Read the model definition and answer for the solid it produces. Units are mm, in the model's axes. Coordinates: 2 decimals unless noted, no trailing zeros. Use one line per item in the form item = value. Start each with the question number.
from build123d import *

# Parameters (mm, degrees)
BASE_FLANGE1_DEPTH = 3.175
SKETCH6_R          = 4.7625
CUT_EXTRUDE1_DEPTH = 140.880281402


# Sheet-metal steps are written as plain solids
with BuildPart() as part:
    # Sketch1 → Base-Flange1 (new body)
    with BuildSketch(Plane(origin=(0, 0, 0), x_dir=(1, 0, 0), z_dir=(0, 1, 0))):
        with BuildLine():
            Line((-69.85, -107.95), (69.85, -107.95))
            ThreePointArc((69.85, -107.95), (83.320384182, -102.370384182), (88.9, -88.9))
            Line((88.9, -88.9), (88.9, 88.9))
            ThreePointArc((88.9, 88.9), (83.320384182, 102.370384182), (69.85, 107.95))
            Line((69.85, 107.95), (-69.85, 107.95))
            ThreePointArc((-69.85, 107.95), (-83.320384182, 102.370384182), (-88.9, 88.9))
            Line((-88.9, 88.9), (-88.9, -88.9))
            ThreePointArc((-88.9, -88.9), (-83.320384182, -102.370384182), (-69.85, -107.95))
        make_face()
    extrude(amount=-BASE_FLANGE1_DEPTH)

    # Sketch6 → Cut-Extrude1 (cut, through all)
    with BuildSketch(Plane(origin=(0, 0, 0), x_dir=(1, 0, 0), z_dir=(0, 1, 0))):
        with Locations(Location((-69.85, -88.9, 0), (0, 0, 270))):
            Circle(SKETCH6_R)
        with Locations(Location((69.85, -88.9, 0), (0, 0, 270))):
            Circle(SKETCH6_R)
        with Locations(Location((69.85, 88.9, 0), (0, 0, 270))):
            Circle(SKETCH6_R)
        with Locations(Location((-69.85, 88.9, 0), (0, 0, 270))):
            Circle(SKETCH6_R)
    extrude(amount=-CUT_EXTRUDE1_DEPTH, mode=Mode.SUBTRACT)


solid = part.part
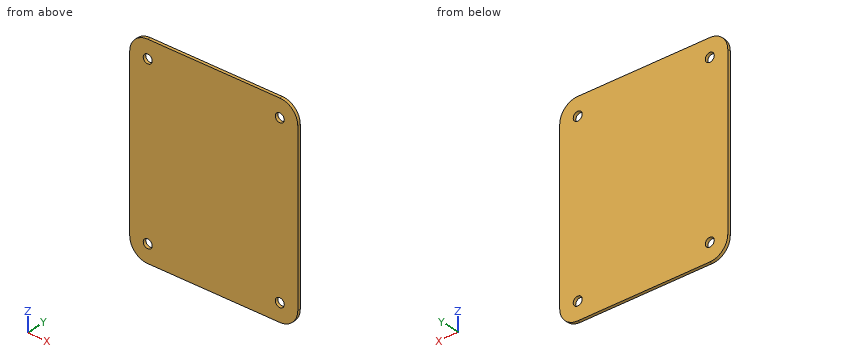
Q1. Given P1, Ø1.5, axis at x = -69, z = 72.5, coming from the +Y side, flat-ended and moving along its own axis, determine where the tip first touches the part or whether it passes through.
Q2. A cutting plane is placed at A-A (y = -0.9). Give the number of separate pieces and of enclosed holes in the cut face, then the cut area to 3 significant figures.
Q3. Consider probe 1 along X at (y, z) = (-1.85, 88.9); probe 2 along X at (y, z) = (-0.65, -86); probe 3 along Z at (x, y) = (-77.5, -0.9). Determine where each line is inside the solid, lowest interval first.
Result sheet:
q1.P1 = 0
q2.separate_pieces = 1
q2.enclosed_holes = 4
q2.area = 37,800 mm^2
q3.probe_1 = -88.9 to -74.61, -65.09 to 65.09, 74.61 to 88.9
q3.probe_2 = -88.9 to -73.63, -66.07 to 66.07, 73.63 to 88.9
q3.probe_3 = -106.35 to 106.35
